Source: three-view drawing plus pictorial views. Frame: mm from the lowest corner of the part. A direction names the side the tool comes from. Coordinates: 2 decimals unless noted, no trailing zeros. Loops run counter-clockwise (first coordinate to the right, second up) from the corner with the lowest first, then second, coordinate; pieces in that order, holes last. Notation, with made-up numbers: M 11.25,-10.75 L 24.25,-10.75 A20 ccw 24.25,5.25 Z; hole C 60.25,9 d2. An arc over 180 degrees is marked long. Use a Markdown table: item, result. Add a question column.
1. Pin query (flat end, axial travel): pin 1 (2 mm diameter, centred on x = 2.5, y = 4.5, fed in from +Z); pin 2 (2 mm diameter, centred on x = 5.5, y = 10, fed in from -Z); pin 3 (2 mm diameter, centred on x = 6.5, y = 3, fed in from +Z). Return the tip coordinate at first contact, or that it passes through.
2. Section B-B on z = 6.5. Output: boundary loops of the cut face in (x, y), then the cut area to 3 significant figures.
3. Section C-C on y = 3. Output: boundary loops of the cut face in (x, z).
4. Set-up query: the marked faces 1, 2, 3 and 4. Return all of +Z, -Z, +X, -X, +Y, -Y with unobstructed straight access to the full face (end or side cutting, diameter ignored); none if empty.
5. Line query: L1, parallel to Y at x = 12.1, z = 6.5; L2, parallel to Y at x = 5.5, z = 1.5; L3, parallel to X at y = 8.75, z = 6.5. Output: solid intervals per line, ascending. Write a range as [from, to].
6. Draft query along Y for the marked faces 5, 6 and 7. Return one class per face: +Y half, -Y half, draft (parallel to the pull), parting line (faces both ways), or undercut.
7. Section D-D on z = 1. Output: boundary loops of the cut face in (x, y), then the cut area to 3 significant figures.
8. Section A-A on x = 6.5. Output: boundary loops of the cut face in (y, z).
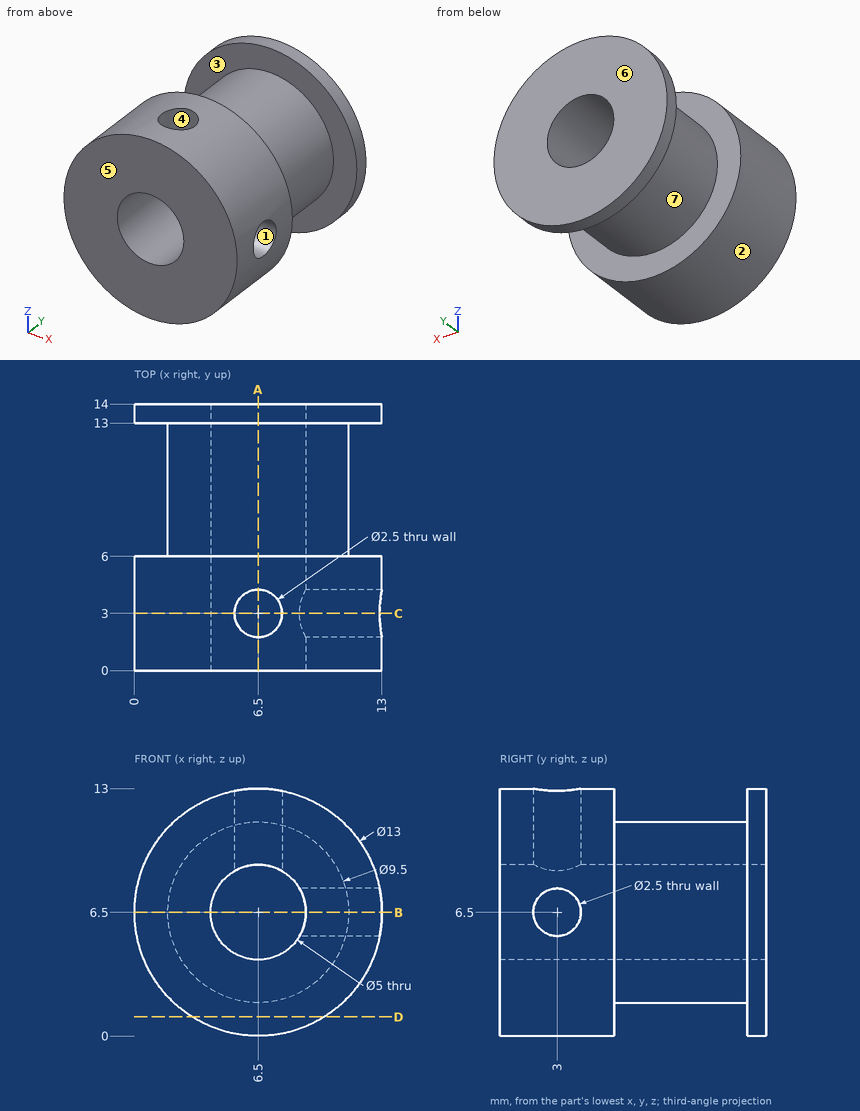
Answers below:
| question | item | result |
|---|---|---|
| 1 | pin 1 | stops at z = 12.27 |
| 1 | pin 2 | stops at z = 1.75 |
| 1 | pin 3 | stops at z = 4.21 |
| 2 | outline | M 0,0 L 4,0 L 4,14 L 0,14 L 0,13 L 1.75,13 L 1.75,6 L 0,6 Z; M 9,0 L 13,0 L 13,1.75 L 9,1.75 Z; M 9,4.25 L 13,4.25 L 13,6 L 11.25,6 L 11.25,13 L 13,13 L 13,14 L 9,14 Z |
| 2 | area | 77.5 mm² |
| 3 | outline | M 5.25,8.67 L 5.25,12.88 A6.5 ccw long 12.88,5.25 L 8.67,5.25 A2.5 cw long Z; M 7.75,8.67 A2.5 cw 8.67,7.75 L 12.88,7.75 A6.5 ccw 7.75,12.88 Z |
| 4 | face 1 | +X |
| 4 | face 2 | +Y, -Y |
| 4 | face 3 | none |
| 4 | face 4 | +Z |
| 5 | L1 | y = [0, 1.75], [4.25, 6], [13, 14] |
| 5 | L2 | y = [0, 6], [13, 14] |
| 5 | L3 | x = [1.75, 4], [9, 11.25] |
| 6 | face 5 | -Y half |
| 6 | face 6 | +Y half |
| 6 | face 7 | undercut |
| 7 | outline | M 3.04,0 L 9.96,0 L 9.96,6 L 3.04,6 Z; M 3.04,13 L 9.96,13 L 9.96,14 L 3.04,14 Z |
| 7 | area | 48.5 mm² |
| 8 | outline | M 0,0 L 6,0 L 6,1.75 L 13,1.75 L 13,0 L 14,0 L 14,4 L 0,4 Z; M 0,9 L 1.75,9 L 1.75,13 L 0,13 Z; M 4.25,9 L 14,9 L 14,13 L 13,13 L 13,11.25 L 6,11.25 L 6,13 L 4.25,13 Z |
